```python
from build123d import *

# Parameters (mm, degrees)
EXTRUDE_THIN1_DEPTH = 673.1
CUT_EXTRUDE2_DEPTH  = 677.1


with BuildPart() as part:
    # Sketch1 → Extrude-Thin1 (new body, symmetric)
    with BuildSketch(Plane.XY):
        with BuildLine():
            Line((-336.55, 1067.077736577), (-336.55, 1114.454951942))
            ThreePointArc((-336.55, 1114.454951942), (-335.785416867, 1117.475815795), (-333.675789474, 1119.769214594))
            ThreePointArc((-333.675789474, 1119.769214594), (-174.087631358, 1193.813707994), (0, 1219.2))
            Line((0, 1219.2), (0, 1220.7))
            ThreePointArc((0, 1220.7), (-174.515996593, 1195.251241724), (-334.496842105, 1121.024552228))
            ThreePointArc((-334.496842105, 1121.024552228), (-337.104806678, 1118.189405682), (-338.05, 1114.454951942))
            Line((-338.05, 1114.454951942), (-338.05, 1067.077736577))
            Line((-338.05, 1067.077736577), (-336.55, 1067.077736577))
        make_face()
    extrude_thin1 = extrude(amount=EXTRUDE_THIN1_DEPTH, both=True)

    # Mirror1: Extrude-Thin1 across plane
    add(extrude_thin1.mirror(Plane(origin=(0, 0, 0), x_dir=(0, 0, 1), z_dir=(1, 0, 0))))

    # Sketch3 → Cut-Extrude2 (cut, through all)
    with BuildSketch(Plane.ZY.offset(338.05)):
        with BuildLine():
            Line((508, 1092.2), (508, 1067.077736577))
            Line((508, 1067.077736577), (520.7, 1067.077736577))
            Line((520.7, 1067.077736577), (520.7, 1092.2))
            ThreePointArc((520.7, 1092.2), (514.35, 1098.55), (508, 1092.2))
        make_face()
        with BuildLine():
            Line((-520.7, 1067.077736577), (-508, 1067.077736577))
            Line((-508, 1067.077736577), (-508, 1092.2))
            ThreePointArc((-508, 1092.2), (-514.35, 1098.55), (-520.7, 1092.2))
            Line((-520.7, 1092.2), (-520.7, 1067.077736577))
        make_face()
    extrude(amount=-CUT_EXTRUDE2_DEPTH, mode=Mode.SUBTRACT)


solid = part.part
```
Geometry: final body of the model. Coordinates: model frame, mm. Coordinates: 2 decimals unless noted, no trailing zeros. Order: outer loops, then holes, each group sorted by start corner. A loop starts at its lowest first (then second) coordinate and runs counter-clockwise, first axis right, second up. Notation, with made-up numbers: (37, 36) - (92, 36) arc R18 ccw to (92, 43) - close; hole circle Ø5 at (20, 15.5). An arc over 180 degrees is marked (long way). Write each question's results on one line, items separated by ' | '.
1) Pull-direction query (X, two-part tool) for faces 1 (the flat face through (-336.55, 1090, 9)), 2 (the flat face through (338.05, 1091, 9)), 3 (the flat face through (-338.05, 1091, 9)); classes: pulls with the +X half, pulls with the -X half, needs draft (parallel to the pull), parting line crosses it, or undercut.
Results list:
face 1: undercut | face 2: pulls with the +X half | face 3: pulls with the -X half
2) Section C-C, the plane x = 189. Return loops of the section in (y, z), plus the area to 3 significant figures.
Results list:
outline: (1189.16, -673.1) - (1190.74, -673.1) - (1190.74, 673.1) - (1189.16, 673.1) - close | area: 2,120 mm^2
3) Section A-A, the plane z = 450. Return loops of the section in (x, y).
Results list:
outline: (-338.05, 1067.08) - (-336.55, 1067.08) - (-336.55, 1114.45) arc R6.35 cw to (-333.68, 1119.77) arc R609.6 cw to (333.68, 1119.77) arc R6.35 cw to (336.55, 1114.45) - (336.55, 1067.08) - (338.05, 1067.08) - (338.05, 1114.45) arc R7.85 ccw to (334.5, 1121.02) arc R611.1 ccw to (-334.5, 1121.02) arc R7.85 ccw to (-338.05, 1114.45) - close
4) Pin query (flat end, axial travel): pin 1 (12 mm diameter, centred on y = 1132, z = 342.5, fed in from -X); pin 2 (3 mm diameter, centred on y = 1142, z = -472, fed in from -X); pin 3 (3 mm diameter, centred on y = 1123, z = -52, fed in from +X). Return the tip coordinate at first contact, or that it passes through.
Results list:
pin 1: x = -326.76 | pin 2: x = -302.64 | pin 3: x = 333.77
5) Line query: line 1 (X direction, y = 1107.5, z = 593); line 2 (X direction, y = 1120.5, z = -347.5); line 3 (Y direction, x = -188.5, z = -73.5). Output: solid intervals per line, ascending. Write a range as from..to.
Results list:
line 1: -338.05..-336.55, 336.55..338.05 | line 2: -335.21..-332.56, 332.56..335.21 | line 3: 1189.32..1190.9
6) Section D-D, the plane x = 291. Return loops of the section in (y, z).
Results list:
outline: (1145.26, -673.1) - (1146.97, -673.1) - (1146.97, 673.1) - (1145.26, 673.1) - close
